```python
from build123d import *
from build123d.topology import SkipClean

# Parameters (mm, degrees)
EXTRUDE_1_DEPTH          = 3
EXTRUDE_1_DEPTH_BACK     = 3
SKETCH_1_R               = 1.025
SKETCH_1_R_2             = 2.6
CUT_EXTRUDE_1_DEPTH      = 10
CUT_EXTRUDE_1_DEPTH_BACK = 10
SKETCH_3_W               = 15
SKETCH_3_H               = 3
SKETCH_3_H_2             = 1.5
FILLET_1_R               = 3
SKETCH_4_R               = 4
SKETCH_4_R_2             = 2.6
EXTRUDE_2_DEPTH          = 0.5
EXTRUDE_START            = 0.5
SKETCH_5_R               = 2.6
EXTRUDE_3_DEPTH          = 0.5
SKETCH_6_R               = 1.2
CUT_EXTRUDE_2_DEPTH      = 2
SCALE_1_SCALE            = 0.6


with BuildPart() as part:
    # Sketch 1 → Extrude 1 (new, two sides: drawn at the far end of the back side and taken through both)
    with BuildSketch(Plane.XY.offset(-EXTRUDE_1_DEPTH_BACK)):
        with BuildLine():
            Line((-21, 4), (12, 4))
            ThreePointArc((12, 4), (16, 0), (12, -4))
            Line((12, -4), (-21, -4))
            ThreePointArc((-21, -4), (-25, 0), (-21, 4))
        make_face()
        with Locations((-21, 0)):
            Circle(SKETCH_1_R, mode=Mode.SUBTRACT)
        with Locations((12, 0)):
            Circle(SKETCH_1_R_2, mode=Mode.SUBTRACT)
    extrude(amount=EXTRUDE_1_DEPTH + EXTRUDE_1_DEPTH_BACK)

    # Sketch 3 → Cut-Extrude 1 (cut, two sides: drawn at the far end of the back side and taken through both)
    with BuildSketch(Plane(origin=(0, 0, 0), x_dir=(1, 0, 0), z_dir=(0, 1, 0)).offset(-CUT_EXTRUDE_1_DEPTH_BACK)):
        with Locations((-17.5, 0)):
            Rectangle(SKETCH_3_W, SKETCH_3_H)
        with Locations((8.5, 2.25)):
            Rectangle(SKETCH_3_W, SKETCH_3_H_2)
        with Locations((8.5, -2.25)):
            Rectangle(SKETCH_3_W, SKETCH_3_H_2)
    extrude(amount=CUT_EXTRUDE_1_DEPTH + CUT_EXTRUDE_1_DEPTH_BACK, mode=Mode.SUBTRACT)

    # Fillet 1
    fillet_1_edges = [part.edges().sort_by_distance(p)[0] for p in [
        (1, 4, 2.25),
        (1, -4, 2.25),
        (1, 4, -2.25),
        (1, -4, -2.25),
    ]]
    fillet(fillet_1_edges, radius=FILLET_1_R)

    # Sketch 4 → Extrude 2 (add)
    with SkipClean():  # the faces are left unmerged after this step: merging them gives an invalid solid
        with BuildSketch(Plane.XY.offset(1.5)):
            with Locations((12, 0)):
                Circle(SKETCH_4_R)
            with Locations((12, 0)):
                Circle(SKETCH_4_R_2, mode=Mode.SUBTRACT)
        extrude(amount=EXTRUDE_2_DEPTH)
    add(part.part.scale(1), mode=Mode.REPLACE)  # the faces are merged on a copy

    # Sketch 5 → Extrude 3 (add)
    with BuildSketch(Plane(origin=(0, 0, -1.5), x_dir=(-1, 0, 0), z_dir=(0, 0, -1)).offset(EXTRUDE_START)):
        with BuildLine():
            ThreePointArc((-12, 4), (-16, 0), (-12, -4))
            ThreePointArc((-12, -4), (-8, 0), (-12, 4))
        make_face()
        with Locations(Location((-12, 0, 0), (0, 0, 180))):
            Circle(SKETCH_5_R, mode=Mode.SUBTRACT)
    extrude(amount=-EXTRUDE_3_DEPTH)

    # Sketch 6 → Cut-Extrude 2 (cut)
    with BuildSketch(Plane.XY.offset(3)):
        with Locations((-21, 0)):
            Circle(SKETCH_6_R)
    extrude(amount=-CUT_EXTRUDE_2_DEPTH, mode=Mode.SUBTRACT)


with BuildPart() as part_1:
    # Scale 1: scaled about (0, 0, 0)
    add(part.part.scale(SCALE_1_SCALE))


solid = part_1.part
```
Check sheet for the modelled part. Datum: model origin and axes. Units: mm. A direction names the side the tool comes from. Give positions to 0.01 mm unless a question says otherwise; leave off trailing zeros. Write each loop counter-clockwise with the first axis right and the second up, starting at its lowest first coordinate (ties: lowest second). Pieces come first, ordered by that corner, then holes. Notation, with made-up numbers: (36.25, 28.5) - (83.25, 28.5) arc R30 ccw to (83.25, 65.5) - close; hole circle Ø10 at (-27, -29). An arc over 180 degrees is marked (long way). Answer as a JSON object with one key per item and string values. Group by question number.
1) Access from +Z, -Z, +X, -X, +Y, -Y to the whole of each face (thin tool, end or side, straight path). Record for faces 1 (the face through (0.059, -1.887, -1.356)), 2 (the face through (0.059, 1.887, -1.344)), 3 (the face through (0.059, 1.887, 1.356)), 4 (the face through (0.059, -1.887, 1.344)).
2) Thickness scan on probe 1 along Y at (x, z) = (7.2, -0.95); probe 2 along Z at (x, y) = (-9.75, 1.1); probe 3 along X at (y, z) = (0, 0.4). Record the ranges inside material, lowest first. Write a range as from..to.
3) Release check for a two-part mould opening along X. For faces 5 (the face through (-11, 0, -0.9)), 6 (the face through (-15, -0.05, -1.36)), 7 (the face through (3, 0, 0.9)) record: pulls with the +X half, pulls with the -X half, needs draft (parallel to the pull), parting line crosses it, or undercut.
4) Sectioned sample at D-D (y = 1.15). Record the cut outline in (x, z).
5) Depth check by flat-ended pin: P1, Ø1.4, axis at y = 1, z = 0, coming from the -X side; P2, Ø1.3, axis at x = -12.6, y = 0, coming from the +Z side; P3, Ø1.4, axis at x = 8, y = 1, coming from the -Z side; P4, Ø2, axis at x = -12, z = -0.5, coming from the +Y side. Enter the tip coordinate at first touch or a pass-through.
6) Sectioned sample at A-A (y = 0). Record the cut outline in (x, z) (3 decimals), then the cut area to 3 significant figures.
7) Sectioned sample at C-C (z = 0.05). Record the cut outline in (x, y).
8) Sectioned sample at B-B (x = -9). Record the cut outline in (y, z).
Geometry results:
{
 "1": {"face 1": "-Z, -Y", "face 2": "-Z, +Y", "face 3": "+Z, +Y", "face 4": "+Z, -Y"},
 "2": {"probe 1": "y = -2.4..-1.56, 1.56..2.4", "probe 2": "z = -1.8..-0.9, 0.9..1.8", "probe 3": "x = -6..5.64, 8.76..9.6"},
 "3": {"face 5": "needs draft", "face 6": "pulls with the -X half", "face 7": "undercut"},
 "4": {"outline": "(-14.71, -1.8) - (0.51, -1.8) - (0.51, -0.9) - (5.09, -0.9) - (5.09, -1.2) - (6.15, -1.2) - (6.15, 1.2) - (5.09, 1.2) - (5.09, 0.9) - (0.51, 0.9) - (0.51, 1.8) - (-14.71, 1.8) - (-14.71, 0.9) - (-6, 0.9) - (-6, -0.9) - (-14.71, -0.9) - close; (8.25, -1.2) - (9.31, -1.2) - (9.31, 1.2) - (8.25, 1.2) - close"},
 "5": {"P1": "stops at x = -6", "P2": "stops at z = -0.9", "P3": "stops at z = -1.2", "P4": "stops at y = 2.4"},
 "6": {"outline": "(-15, -1.8) - (-13.215, -1.8) - (-13.215, -0.9) - (-15, -0.9) - close; (-15, 0.9) - (-13.32, 0.9) - (-13.32, 1.8) - (-15, 1.8) - close; (-11.985, -1.8) - (0.6, -1.8) - (0.6, -0.9) - (4.8, -0.9) - (4.8, -1.2) - (5.64, -1.2) - (5.64, 1.2) - (4.8, 1.2) - (4.8, 0.9) - (0.6, 0.9) - (0.6, 1.8) - (-11.88, 1.8) - (-11.88, 0.9) - (-6, 0.9) - (-6, -0.9) - (-11.985, -0.9) - close; (8.76, -1.2) - (9.6, -1.2) - (9.6, 1.2) - (8.76, 1.2) - close", "area": "49.1 mm^2"},
 "7": {"outline": "(-6, -2.4) - (7.2, -2.4) arc R2.4 ccw to (7.2, 2.4) - (-6, 2.4) - close; hole circle Ø3.12 at (7.2, 0)"},
 "8": {"outline": "(-2.4, -1.8) - (2.4, -1.8) - (2.4, -0.9) - (-2.4, -0.9) - close; (-2.4, 0.9) - (2.4, 0.9) - (2.4, 1.8) - (-2.4, 1.8) - close"}
}
